For this review, take the finished solid that the model builds, in its own axes (mm). Face numbers are marked on the shaded views. A direction names the side the tool comes from. Give positions to 0.01 mm unless a question says otherwise; leave off trailing zeros. Loops run counter-clockwise (first coordinate to the right, second up) from the corner with the lowest first, then second, coordinate; pieces in that order, holes last. Notation, with made-up numbers: (40, 83) - (56, 83) arc R11 cw to (56, 95) - close; hole circle Ø3 at (16, 35.25). An arc over 180 degrees is marked (long way). Put each result on its own line as item: value. Start each with the question number.
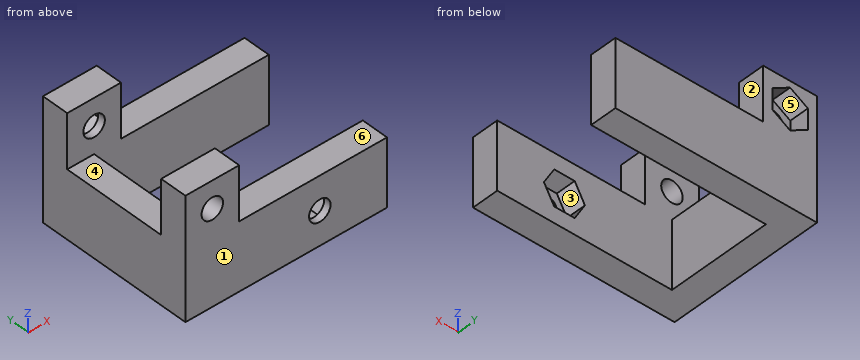
from build123d import *

# Parameters (mm, degrees)
SALIENTE_EXTRUIR1_DEPTH = 10
CORTAR_EXTRUIR2_REACH   = 6
CROQUIS3_R              = 1.6
CORTAR_EXTRUIR3_DEPTH   = 2.95
CROQUIS6_W              = 8
CROQUIS6_H              = 4
SALIENTE_EXTRUIR2_DEPTH = 8
CORTAR_EXTRUIR4_DEPTH   = 2.9
CROQUIS8_R              = 1.6
CORTAR_EXTRUIR5_DEPTH   = 24.5


with BuildPart() as part:
    # Croquis1 → Saliente-Extruir1 (new body)
    with BuildSketch(Plane.XY):
        Polygon((0, 0), (-30, 0), (-30, -23.5), (0, -23.5), (0, -19.5), (-26, -19.5), (-26, -4), (0, -4), align=None)
    extrude(amount=SALIENTE_EXTRUIR1_DEPTH)

    # Croquis3 → Cortar-Extruir2 (cut, up to next)
    with BuildSketch(Plane(origin=(0, -19.5, 0), x_dir=(1, 0, 0), z_dir=(0, 1, 0)), mode=Mode.PRIVATE) as cortar_extruir2_sk1:
        with Locations((-10, -5)):
            Circle(CROQUIS3_R)
    cortar_extruir2_tool1 = extrude(cortar_extruir2_sk1.sketch, amount=-CORTAR_EXTRUIR2_REACH, mode=Mode.PRIVATE) & part.part
    add(cortar_extruir2_tool1.solids().sort_by_distance((-10, -19.5, 5))[0], mode=Mode.SUBTRACT)

    # Croquis5 → Cortar-Extruir3 (cut)
    with BuildSketch(Plane(origin=(0, -19.5, 0), x_dir=(1, 0, 0), z_dir=(0, 1, 0))):
        Polygon((-8.475, -7.641377482), (-6.95, -5), (-8.475, -2.358622518), (-11.525, -2.358622518), (-13.05, -5), (-11.525, -7.641377482), align=None)
    extrude(amount=-CORTAR_EXTRUIR3_DEPTH, mode=Mode.SUBTRACT)

    # Croquis6 → Saliente-Extruir2 (add)
    with BuildSketch(Plane.XY.offset(10)):
        with Locations((-26, -2)):
            Rectangle(CROQUIS6_W, CROQUIS6_H)
        with Locations((-26, -21.5)):
            Rectangle(CROQUIS6_W, CROQUIS6_H)
    extrude(amount=SALIENTE_EXTRUIR2_DEPTH)

    # Croquis7 → Cortar-Extruir4 (cut)
    with BuildSketch(Plane(origin=(0, 0, 0), x_dir=(1, 0, 0), z_dir=(0, 1, 0))):
        Polygon((-26, -17.05), (-23.358622518, -15.525), (-23.358622518, -12.475), (-26, -10.95), (-28.641377482, -12.475), (-28.641377482, -15.525), align=None)
    extrude(amount=-CORTAR_EXTRUIR4_DEPTH, mode=Mode.SUBTRACT)

    # Croquis8 → Cortar-Extruir5 (cut, through all)
    with BuildSketch(Plane(origin=(0, 0, 0), x_dir=(1, 0, 0), z_dir=(0, 1, 0))):
        with Locations((-26, -14)):
            Circle(CROQUIS8_R)
    extrude(amount=-CORTAR_EXTRUIR5_DEPTH, mode=Mode.SUBTRACT)


solid = part.part
1) Wall thickness on probe 1 along Y at (x, z) = (-16.75, 2.75); probe 2 along Z at (x, y) = (-26, -20.85); probe 3 along X at (y, z) = (-3.45, 14): over which ranges is each line inside the solid? List them lowest first.
2) Take a section at B-B on x = -10. State the section outline as (y, z) points, and give its area (3 significant figures).
3) Machinability: for the marked faces 4, 5 and 6, which of the approach directions +Z, -Z, +X, -X, +Y, -Y give a long, thin tool a straight path to every point of the face, cutting with its end or side? Answer none if there is none.
4) Mouldability with a two-part tool opening along X and no side actions: class the marked faces 1, 2 and 3 as released by +X, released by -X, zero draft, split by the parting line, or undercut.
5) Take a section at D-D on x = -19. State the section outline as (y, z) points, and give its area (3 significant figures).
6) Insertion check: P1, Ø2, axis at x = -27, y = -13, coming from the +Z side; P2, Ø2.5, axis at y = -1, z = 14.5, coming from the +X side; P3, Ø9, axis at x = -17, z = 12.5, coming from the +Y side. Each pin has a flat end and moves straight along its axis. Give the tip position at first contact, or say it passes through.
7) Take a section at A-A on y = -3.5. State the section outline as (x, z) points.
8) Take a section at C-C on z = 14. State the section outline as (x, y) points, and give its area (3 significant figures).
Answers follow:
1. probe 1: -23.5 to -19.5, -4 to 0
1. probe 2: 0 to 12.4, 15.6 to 18
1. probe 3: -30 to -27.6, -24.4 to -22
2. outline: (-23.5, 0) - (-19.5, 0) - (-19.5, 2.36) - (-22.45, 2.36) - (-22.45, 3.4) - (-23.5, 3.4) - close; (-23.5, 6.6) - (-22.45, 6.6) - (-22.45, 7.64) - (-19.5, 7.64) - (-19.5, 10) - (-23.5, 10) - close; (-4, 0) - (0, 0) - (0, 10) - (-4, 10) - close
2. area: 61.1 mm2
3. face 4: +Z, +X, -X
3. face 5: +Y
3. face 6: +Z, +X, +Y, -Y
4. face 1: zero draft
4. face 2: released by +X
4. face 3: undercut
5. outline: (-23.5, 0) - (-19.5, 0) - (-19.5, 10) - (-23.5, 10) - close; (-4, 0) - (0, 0) - (0, 10) - (-4, 10) - close
5. area: 80.0 mm2
6. P1: z = 10
6. P2: x = -22
6. P3: y = 0
7. outline: (-30, 0) - (0, 0) - (0, 10) - (-22, 10) - (-22, 18) - (-30, 18) - close; hole circle Ø3.2 at (-26, 14)
8. outline: (-30, -23.5) - (-27.6, -23.5) - (-27.6, -19.5) - (-30, -19.5) - close; (-30, -4) - (-27.6, -4) - (-27.6, -2.9) - (-28.64, -2.9) - (-28.64, 0) - (-30, 0) - close; (-24.4, -23.5) - (-22, -23.5) - (-22, -19.5) - (-24.4, -19.5) - close; (-24.4, -4) - (-22, -4) - (-22, 0) - (-23.36, 0) - (-23.36, -2.9) - (-24.4, -2.9) - close
8. area: 32.4 mm2
